Geometry: final body of the model. Coordinates: model frame, mm. Face numbers are marked on the shaded views. A direction names the side the tool comes from. Round coordinates to 2 decimals unless told otherwise and drop trailing zeros. Loops run counter-clockwise (first coordinate to the right, second up) from the corner with the lowest first, then second, coordinate; pieces in that order, holes last. Notation, with made-up numbers: (-29.75, 17) - (-16.75, 17) arc R27 ccw to (-16.75, 55) - close; hole circle Ø5 at (41.5, -22). An arc over 180 degrees is marked (long way). Answer as CSV lines item,"result".
from build123d import *

# Parameters (mm, degrees)
F1_DEPTH = 10
F2_SIZE  = 0.5


# Not quite as in the source:
# - ends of sketch curves that miss each other by under 0.0002 mm in the source are joined


with BuildPart() as f1:
    # F0 (on Top) → F1 (new body)
    with BuildSketch(Plane.XY):
        with BuildLine():
            Line((3.3542521534, 2.75), (-3.3557469528, 2.75))
            ThreePointArc((-3.3557469528, 2.75), (-6.1057473997, -4.469e-07), (-3.3557469528, -2.7500008938))
            Line((-3.3557469528, -2.7500008938), (3.3542521534, -2.75))
            ThreePointArc((3.3542521534, -2.75), (6.1042526003, -4.469e-07), (3.3542521534, 2.75))
        make_face()
        with BuildLine():
            Line((-3.3557469528, 1.25), (3.3542521534, 1.25))
            ThreePointArc((3.3542521534, 1.25), (4.6042523768, 0.000746953), (3.3557469528, -1.25))
            Line((3.3557469528, -1.25), (-3.3542521534, -1.25))
            ThreePointArc((-3.3542521534, -1.25), (-4.6057471763, -0.0007478467), (-3.3557469528, 1.25))
        make_face(mode=Mode.SUBTRACT)
    extrude(amount=F1_DEPTH)

    # F2
    f2_edges = [f1.edges().sort_by_distance(p)[0] for p in [
        (-0.000747, -2.75, 10),
        (6.104253, 0, 10),
        (-0.000747, 2.75, 10),
        (-6.105747, 0, 10),
        (-0.000747, 1.25, 10),
        (4.604252, 0.000747, 10),
        (0.000747, -1.25, 10),
        (-4.605747, -0.000748, 10),
        (-0.000747, -2.75, 0),
        (6.104253, 0, 0),
        (-0.000747, 2.75, 0),
        (-6.105747, 0, 0),
        (-0.000747, 1.25, 0),
        (4.604252, 0.000747, 0),
        (0.000747, -1.25, 0),
        (-4.605747, -0.000748, 0),
    ]]
    chamfer(f2_edges, length=F2_SIZE)


solid = f1.part
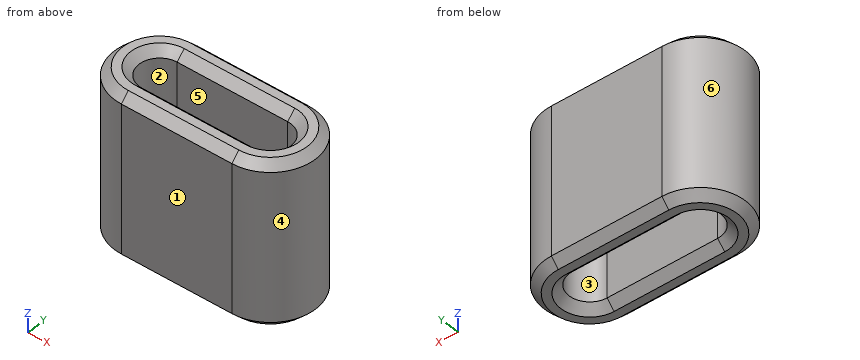
(1) Draft query along X for the marked faces 3, 4, 5 and 6. Return one class per face: pulls with the +X half, pulls with the -X half, needs draft (parallel to the pull), parting line crosses it, or undercut.
Findings below:
face 3,"undercut"
face 4,"pulls with the +X half"
face 5,"undercut"
face 6,"pulls with the -X half"
(2) Section A-A (x = -3). Output: boundary loops of the cut face in (y, z).
Findings below:
outline,"(-2.75, 0.5) - (-2.25, 0) - (-1.75, 0) - (-1.25, 0.5) - (-1.25, 9.5) - (-1.75, 10) - (-2.25, 10) - (-2.75, 9.5) - close; (1.25, 0.5) - (1.75, 0) - (2.25, 0) - (2.75, 0.5) - (2.75, 9.5) - (2.25, 10) - (1.75, 10) - (1.25, 9.5) - close"
(3) Section B-B (z = 2.5). Output: boundary loops of the cut face in (x, y).
Findings below:
outline,"(-3.36, -2.75) - (3.35, -2.75) arc R2.75 ccw to (3.35, 2.75) - (-3.36, 2.75) arc R2.75 ccw to start; hole (-3.36, 1.25) arc R1.25 ccw to (-3.35, -1.25) - (3.36, -1.25) arc R1.25 ccw to (3.35, 1.25) - close"
(4) Material intervals for line 1 along Y through (x, z) = (-0.25, 9); line 2 along Y through (x, z) = (-4.25, 2.5); line 3 along X through (y, z) = (-0.4, 7) (1 decimal), sorted ascending.
Findings below:
line 1,"-2.75 to -1.25, 1.25 to 2.75"
line 2,"-2.6 to -0.87, 0.87 to 2.6"
line 3,"-6.1 to -4.5, 4.5 to 6.1"
(5) Access query for the marked faces 1 and 2. Directions: +Z, -Z, +X, -X, +Y, -Y. A direction counts if a zero-diameter tool reaches every point of the face in a straight line with its end or side. Return the directions, or none.
Findings below:
face 1,"+Z, -Z, +X, -X, -Y"
face 2,"+Z, -Z"
